Autodesk Inventor part; units mm, degrees
ref_plane "YZ Plane" through (0, 0, 0) normal (1, 0, 0) x (0, 1, 0)
ref_plane "XZ Plane" through (0, 0, 0) normal (0, 1, 0) x (-1, 0, 0)
ref_plane "XY Plane" through (0, 0, 0) normal (0, 0, 1) x (1, 0, 0)
sketch "Sketch_20" plane through (0, 0, 0) normal (1, 0, 0) x (0, 1, 0)
  line L0 (19.5, -14.1) -> (11.5, -14.1)
  line L1 (11.5, -14.1) -> (11.5, -22.5)
  line L2 (11.5, -22.5) -> (17.5, -22.5)
  arc A0 (17.5, -22.5) -> (19.5, -20.5) centre (17.5, -20.5) ccw
  line L3 (19.5, -20.5) -> (19.5, -14.1)
extrude "Extrusion1" add sketch "Sketch_20" along normal mid plane 8
sketch "Sketch_2" plane through (0, 0, 0) normal (0, 0, 1) x (1, 0, 0)
  line L0 (-10, 5) -> (10, 5)
  line L1 (10, 5) -> (10, 25)
  line L2 (10, 25) -> (-10, 25)
  line L3 (-10, 25) -> (-10, 5)
  line L4 (-4, 11.5) -> (4, 11.5)
  line L5 (4, 11.5) -> (4, 17.5)
  arc A0 (4, 17.5) -> (2, 19.5) centre (2, 17.5) ccw
  line L6 (2, 19.5) -> (-2, 19.5)
  arc A1 (-2, 19.5) -> (-4, 17.5) centre (-2, 17.5) ccw
  line L7 (-4, 17.5) -> (-4, 11.5)
extrude "Extrusion2" cut sketch "Sketch_2" along normal mid plane 57
sketch "Sketch_13" plane through (0, 0, 0) normal (0, 1, 0) x (-1, 0, 0)
  line L0 (10, -10) -> (-10, -10)
  line L1 (-10, -10) -> (-10, -25)
  line L2 (-10, -25) -> (10, -25)
  line L3 (10, -25) -> (10, -10)
  line L4 (4, -20.5) -> (4, -12.5)
  line L5 (4, -12.5) -> (-4, -12.5)
  line L6 (-4, -12.5) -> (-4, -20.5)
  arc A0 (-4, -20.5) -> (-2, -22.5) centre (-2, -20.5) ccw
  line L7 (-2, -22.5) -> (2, -22.5)
  arc A1 (2, -22.5) -> (4, -20.5) centre (2, -20.5) ccw
extrude "Extrusion3" cut sketch "Sketch_13" along normal blind 25
sketch "Sketch_12" plane through (0, 0, 0) normal (1, 0, 0) x (0, 1, 0)
  line L0 (3.4, -18.5) -> (11.5, -18.5)
  line L1 (11.5, -18.5) -> (11.5, -23.4)
  line L2 (11.5, -23.4) -> (8, -23.4)
  line L3 (8, -23.4) -> (8, -23.5)
  line L4 (8, -23.5) -> (7.4226, -24.5)
  line L5 (7.4226, -24.5) -> (6.0774, -24.5)
  line L6 (6.0774, -24.5) -> (5.5, -23.5)
  line L7 (5.5, -23.5) -> (5.5, -22.4)
  line L8 (5.5, -22.4) -> (3.4, -22.4)
  line L9 (3.4, -22.4) -> (3.4, -18.5)
  line L10 (3.4, -18.5) -> (11.5, -18.5)
revolve "Revolution1" add sketch "Sketch_12" angle 360 about axis through (0, 3.4, -18.5) along (0, -1, 0)
sketch "Sketch_6" plane through (0, 0, 0) normal (0, 1, 0) x (-1, 0, 0)
  line L0 (10, -8.5) -> (-10, -8.5)
  line L1 (-10, -8.5) -> (-10, -28.5)
  line L2 (-10, -28.5) -> (10, -28.5)
  line L3 (10, -28.5) -> (10, -8.5)
  line L4 (5, -15.6132) -> (0, -12.7265)
  line L5 (0, -12.7265) -> (-5, -15.6132)
  line L6 (-5, -15.6132) -> (-5, -21.3868)
  line L7 (-5, -21.3868) -> (0, -24.2735)
  line L8 (0, -24.2735) -> (5, -21.3868)
  line L9 (5, -21.3868) -> (5, -15.6132)
extrude "Extrusion4" cut sketch "Sketch_6" along normal blind 10
sketch "Sketch_7" plane through (0, 0, 0) normal (1, 0, 0) x (0, 1, 0)
  line L0 (0, -18.5) -> (3.4, -18.5)
  line L1 (3.4, -18.5) -> (3.4, -21)
  line L2 (3.4, -21) -> (0, -21)
  line L3 (0, -21) -> (0, -18.5)
  line L4 (0, -18.5) -> (3.4, -18.5)
revolve "Revolution2" add sketch "Sketch_7" angle 360 about axis through (0, 0, -18.5) along (0, -1, 0)
thread "Thread1"
sketch "Sketch_15" plane through (0, 0, 0) normal (1, 0, 0) x (0, 1, 0)
  line L0 (15.5, -14.1) -> (15.5, 0)
  line L1 (15.5, 0) -> (20.4, 0)
  arc A0 (20.9, -0.5) -> (20.4, 0) centre (20.4, -0.5) ccw
  line L2 (20.9, -0.5) -> (20.9, -1)
  line L3 (20.9, -1) -> (19.1, -1)
  line L4 (19.1, -1) -> (19.1, -2.6)
  line L5 (19.1, -2.6) -> (21, -2.6)
  line L6 (21, -2.6) -> (21, -3.6)
  line L7 (21, -3.6) -> (21.4, -3.6)
  line L8 (21.4, -3.6) -> (21.4, -14.1)
  line L9 (21.4, -14.1) -> (15.5, -14.1)
  line L10 (15.5, -14.1) -> (15.5, 0)
revolve "Revolution3" add sketch "Sketch_15" angle 360 about axis through (0, 15.5, -14.1) along (0, 0, -1)
sketch "Sketch_18" plane through (0, 0, 0) normal (1, 0, 0) x (0, 1, 0)
  line L0 (15.5, -14.5) -> (15.5, 0)
  line L1 (15.5, 0) -> (18.5, 0)
  line L2 (18.5, 0) -> (18.5, -14.5)
  line L3 (18.5, -14.5) -> (15.5, -14.5)
  line L4 (15.5, -14.5) -> (15.5, 0)
revolve "Revolution4" cut sketch "Sketch_18" angle 360 about axis through (0, 15.5, -14.5) along (0, 0, -1)
properties part number "GWJL6-M5"
Could you check a few things on this model? Use its own coordinates, in mm. A direction names the side the tool comes from. Give positions to 0.01 mm unless a question says otherwise; leave off trailing zeros. Order: outer loops, then holes, each group sorted by start corner. A loop starts at its lowest first (then second) coordinate and runs counter-clockwise, first axis right, second up. Notation, with made-up numbers: M 84,-1 L 110,-1 A16 ccw 110,30 Z; hole C 76,50 d3. An arc over 180 degrees is marked long. One line per question, with ' | ' between items.
1. I want a section at C-C (x = 4.5). Give the number of separate pieces and of enclosed holes in the cut face, and give its area (3 significant figures).
Results:
separate pieces: 3 | enclosed holes: 0 | area: 121 mm²
2. We'd pull the mould along Y, two halves only. Please class faces 1 (the face through (0, 19.5, -17)), 2 (the face through (2.465, 6.733, -14.15)), 3 (the face through (0, 15, -14.5)): +Y half, -Y half, draft (parallel to the pull), parting line (faces both ways), or undercut.
Results:
face 1: +Y half | face 2: draft | face 3: undercut
3. I want a section at D-D (z = -1.75). List the corners of the cut face in (x, y) for me, and give its area (3 significant figures).
Results:
outline: C 0,15.5 d7.2; hole C 0,15.5 d6 | area: 12.4 mm²
4. If I drill on line 1 (X direction, y = 15.5, z = -9.25); line 2 (Y direction, x = -2, z = -15.75); line 3 (X direction, y = 13.75, z = -4.75), over which ranges is the centre line in solid material (lowest first)?
Results:
line 1: -5.9 to -3, 3 to 5.9 | line 2: 3.4 to 19.5 | line 3: -5.63 to -2.44, 2.44 to 5.63
5. I'm going to push flat-ended pins straight in: pin 1 (2 mm diameter, centred on x = 1, y = 16, fed in from -Z); pin 2 (5 mm diameter, centred on x = -1, y = 17, fed in from +Z); pin 3 (1.3 mm diameter, centred on x = -3, z = -14.5, fed in from -Y); pin 4 (3 mm diameter, centred on y = 7, z = -19.5, fed in from +X). Where does each tip first touch, or does it pass through?
Results:
pin 1: z = -22.5 | pin 2: z = 0 | pin 3: y = 5.5 | pin 4: x = 5
6. I want a section at A-A (z = -5). List the corners of the cut face in (x, y) for me, and give its area (3 significant figures).
Results:
outline: C 0,15.5 d11.8; hole C 0,15.5 d6 | area: 81.1 mm²
7. I want a section at B-B (y = 15.5). List the corners of the cut face in (x, z) for me.
Results:
outline: M -5.9,-14.1 L -4,-14.1 L -4,-20.5 A2 ccw -2,-22.5 L 2,-22.5 A2 ccw 4,-20.5 L 4,-14.1 L 5.9,-14.1 L 5.9,-3.6 L 5.5,-3.6 L 5.5,-2.6 L 3.6,-2.6 L 3.6,-1 L 5.4,-1 L 5.4,-0.5 A0.5 ccw 4.9,0 L 3,0 L 3,-14.5 L -3,-14.5 L -3,0 L -4.9,0 A0.5 ccw -5.4,-0.5 L -5.4,-1 L -3.6,-1 L -3.6,-2.6 L -5.5,-2.6 L -5.5,-3.6 L -5.9,-3.6 Z
8. For faces 4 (the face through (0, 20, -14.1)), 5 (the face through (-2.11, 20.58, -3.11)), 6 (the face through (-3.5, 11.5, -14.5)), 7 (the face through (-2.535, 6.733, -14.19)), which set-ups out of +Z, -Z, +X, -X, +Y, -Y let a thin tool reach every point of the face, with its end or its side?
Results:
face 4: none | face 5: +Z | face 6: -X | face 7: +Z, -X, -Y
